For this review, take the finished solid that the model builds, in its own axes (mm). A direction names the side the tool comes from. Round coordinates to 2 decimals unless told otherwise and drop trailing zeros. Order: outer loops, then holes, each group sorted by start corner. A loop starts at its lowest first (then second) coordinate and runs counter-clockwise, first axis right, second up. Notation, with made-up numbers: (-11.5, 26.5) -> (-1.5, 26.5) arc R15 ccw to (-1.5, 32.5) -> close; hole circle Ø4 at (64, -13). An arc over 180 degrees is marked (long way). Answer in a Markdown table with one row per item.
```python
from build123d import *

# Parameters (mm, degrees)
SKETCH1_W           = 10
SKETCH1_H           = 25
BOSS_EXTRUDE1_DEPTH = 25
SKETCH2_W           = 10
SKETCH2_H           = 20
BOSS_EXTRUDE2_DEPTH = 10
CUT_EXTRUDE1_DEPTH  = 40
CUT_EXTRUDE2_DEPTH  = 10
SKETCH5_W           = 15
SKETCH5_H           = 10
BOSS_EXTRUDE3_DEPTH = 10


with BuildPart() as part:
    # Sketch1 → Boss-Extrude1 (new body)
    with BuildSketch(Plane.XY):
        with Locations((5, 12.5)):
            Rectangle(SKETCH1_W, SKETCH1_H)
    extrude(amount=BOSS_EXTRUDE1_DEPTH)

    # Sketch2 → Boss-Extrude2 (add)
    with BuildSketch(Plane(origin=(10, 0, 0), x_dir=(0, 0, -1), z_dir=(1, 0, 0))):
        with Locations((-5, 10)):
            Rectangle(SKETCH2_W, SKETCH2_H)
    extrude(amount=BOSS_EXTRUDE2_DEPTH)

    # Sketch3 → Cut-Extrude1 (cut)
    with BuildSketch(Plane.XY.offset(25)):
        Polygon((10, 25), (0, 20), (0, 25), align=None)
    extrude(amount=-CUT_EXTRUDE1_DEPTH, mode=Mode.SUBTRACT)

    # Sketch4 → Cut-Extrude2 (cut)
    with BuildSketch(Plane(origin=(20, 0, 0), x_dir=(0, 0, -1), z_dir=(1, 0, 0))):
        Polygon((-10, 10), (0, 20), (-10, 20), align=None)
    extrude(amount=-CUT_EXTRUDE2_DEPTH, mode=Mode.SUBTRACT)

    # Sketch5 → Boss-Extrude3 (add)
    with BuildSketch(Plane.ZY):
        with Locations((7.5, 5)):
            Rectangle(SKETCH5_W, SKETCH5_H)
    extrude(amount=BOSS_EXTRUDE3_DEPTH)


solid = part.part
```
Q1. Take a section at B-B, the plane y = 3. Write out the cut boundary in (x, z), then the cut area to 3 significant figures.
Answer key:
| item | result |
|---|---|
| outline | (-10, 0) -> (20, 0) -> (20, 10) -> (10, 10) -> (10, 25) -> (0, 25) -> (0, 15) -> (-10, 15) -> close |
| area | 500 mm^2 |
Q2. Take a section at A-A, the plane z = 5.25. Write out the cut boundary in (x, y), then the cut area to 4 significant figures.
Answer key:
| item | result |
|---|---|
| outline | (-10, 0) -> (20, 0) -> (20, 14.75) -> (10, 14.75) -> (10, 25) -> (0, 20) -> (0, 10) -> (-10, 10) -> close |
| area | 472.5 mm^2 |
Q3. To check wall thickness, follow probe 1 along Z at (x, y) = (10.5, 9.5); probe 2 along Z at (x, y) = (-6.75, 8.25). State the ranges of each line that lie inside material, in increasing order.
Answer key:
| item | result |
|---|---|
| probe 1 | z = 0 to 10 |
| probe 2 | z = 0 to 15 |
Q4. Clearance check with flat-ended pins moving along their axes: pin 1 Ø11 at (x, y) = (17.5, 3.5) entering from +Z; pin 2 Ø4 at (x, z) = (6.5, 10.5) entering from -Y; pin 3 Ø8 at (y, z) = (6.5, 20) entering from -X; pin 4 Ø11 at (x, z) = (-5, 5.5) entering from +Y. State where each tip first meets the part, or that it passes through.
Answer key:
| item | result |
|---|---|
| pin 1 | stops at z = 10 |
| pin 2 | stops at y = 0 |
| pin 3 | stops at x = 0 |
| pin 4 | stops at y = 20.25 |
Q5. Take a section at D-D, the plane z = 10.5. Write out the cut boundary in (x, y), then the cut area to 3 significant figures.
Answer key:
| item | result |
|---|---|
| outline | (-10, 0) -> (10, 0) -> (10, 25) -> (0, 20) -> (0, 10) -> (-10, 10) -> close |
| area | 325 mm^2 |
Q6. Take a section at C-C, the plane x = 2. Write out the cut boundary in (y, z).
Answer key:
| item | result |
|---|---|
| outline | (0, 0) -> (21, 0) -> (21, 25) -> (0, 25) -> close |
Q7. Tool access review of faces 1 (the face through (10, 15, 15)), 2 (the face through (-5, 10, 7)), 3 (the face through (15, 5, 10)), 4 (the face through (-5, 5, 15)): name each direction out of +Z, -Z, +X, -X, +Y, -Y from which nothing blocks a thin tool from reaching the whole face with its end or side.
Answer key:
| item | result |
|---|---|
| face 1 | +Z, +X, +Y |
| face 2 | +Z, -Z, -X, +Y |
| face 3 | +Z, +X, +Y, -Y |
| face 4 | +Z, -X, +Y, -Y |
